Check sheet for the modelled part. Datum: model origin and axes. Units: mm. A direction names the side the tool comes from. Coordinates: 2 decimals unless noted, no trailing zeros. Loops run counter-clockwise (first coordinate to the right, second up) from the corner with the lowest first, then second, coordinate; pieces in that order, holes last.
Autodesk Inventor part; units mm, degrees
ref_plane "YZ Plane" through (0, 0, 0) normal (1, 0, 0) x (0, 1, 0)
ref_plane "XZ Plane" through (0, 0, 0) normal (0, 1, 0) x (-1, 0, 0)
ref_plane "XY Plane" through (0, 0, 0) normal (0, 0, 1) x (1, 0, 0)
sketch "Sketch1" plane through (0, 0, 0) normal (0, 0, 1) x (1, 0, 0)
  arc A0 (37.1972, 10.8951) -> (38.76, 0) centre (0, 0) ccw
  arc A1 (-36.6776, -2.4605) -> (36.6776, -2.4605) centre (0, 0) ccw
  line L0 (-36.76, 0) -> (36.76, 0)
  line L1 (-36.76, 0) -> (37.1972, 0)
  line L2 (36.6776, -2.4605) -> (-36.6776, -2.4605)
  line L3 (-36.76, 0) -> (-38.76, 0)
  line L4 (37.1972, 0) -> (38.76, 0)
  line L5 (0, 0) -> (27.3, 0)
  line L6 (27.3, 0) -> (27.3, -1.7)
  line L7 (27.3, -1.7) -> (0, -1.7)
  line L8 (0, -1.7) -> (0, 0)
  line L9 (-27.3, 0) -> (-27.3, -1.7)
  line L10 (-27.3, -1.7) -> (0, -1.7)
  dimension "d0" = 77.52
  dimension "d1" = 2
extrude "Extrusion1" add sketch "Sketch1" along normal blind 5 contours L3 L0 L9 L10 L7 L6 L1 L4 A0
sketch "Sketch2" plane through (-27.3, -1.7, 0) normal (0, 1, 0) x (1, 0, 0)
  line L0 (54.6, 0) -> (0, 0)
  line L1 (54.6, 0) -> (54.6, -5)
  line L2 (0, 0) -> (0, -5)
  point P0 (27.3, 0)
  point P1 (27.305, -2.3213)
  dimension "d7" = 2.3213
  dimension "d28" = 27.305
hole "Hole1" at (0.005, -1.7, 2.3213) direction (0, -1, 0) diameter 3.81 depth 2.54
sketch "Sketch3" plane through (0, 0, 5) normal (0, 0, 1) x (1, 0, 0)
  arc A0 (2.6516, -28.9347) -> (-2.75, -29.6637) centre (0, -29.6637) ccw
  line L0 (-0.7992, -29.6638) -> (0.7008, -29.6638)
  line L1 (2.6516, -29.6637) -> (2.6516, -38.4638)
  line L2 (2.6516, -38.4638) -> (-2.75, -38.4638)
  line L3 (-2.75, -38.4638) -> (-2.75, -29.6637)
  line L4 (-0.7992, -29.6638) -> (0.7008, -29.6638)
  line L5 (0.7008, -29.6638) -> (0.7008, -33.1638)
  line L6 (0.7008, -33.1638) -> (-0.7992, -33.1638)
  line L7 (-0.7992, -33.1638) -> (-0.7992, -29.6638)
  line L8 (2.6516, -29.6637) -> (2.6516, -28.9347)
  point P0 (0, 0)
  point P1 (-0.0492, -29.6638)
  point P2 (2.6516, -30.3927)
  dimension "d16" = 5.5
  dimension "d17" = 3.5
  dimension "d18" = 1.5
  dimension "d19" = 0.75
extrude "Extrusion2" add sketch "Sketch3" against normal up to surface (5 mm away)
properties part number "Siding Lock"
1) Section check C-C on y = -35. Enter the section's corners in (x, z).
Answer sheet:
outline: (-16.65, 0) - (-11.24, 0) - (-11.24, 5) - (-16.65, 5) - close; (-2.75, 0) - (2.65, 0) - (2.65, 5) - (-2.75, 5) - close; (11.24, 0) - (16.65, 0) - (16.65, 5) - (11.24, 5) - close
2) Section check D-D on z = 2.95. Enter the section's corners in (x, y).
Answer sheet:
outline: (-38.76, 0) arc R38.76 ccw to (38.76, 0) - (27.3, 0) - (27.3, -1.7) - (1.8, -1.7) - (1.8, -2.46) - (36.68, -2.46) arc R36.76 cw to (2.65, -36.66) - (2.65, -28.93) arc R2.75 ccw to (-2.75, -29.66) - (-2.75, -36.66) arc R36.76 cw to (-36.68, -2.46) - (-1.79, -2.46) - (-1.79, -1.7) - (-27.3, -1.7) - (-27.3, 0) - close; hole (-0.8, -33.16) - (0.7, -33.16) - (0.7, -29.66) - (-0.8, -29.66) - close
3) Mould release check, pull along X, two halves, no side actions. Record for faces 5 (the cylindrical face through (-25.835, -26.15, 2.465)), 6 (the flat face through (33, 0, 2)), 7 (the flat face through (0, -29.664, 3)): +X half, -X half, draft (parallel to the pull), parting line (faces both ways), or undercut.
Answer sheet:
face 5: undercut
face 6: draft
face 7: undercut
4) Section check A-A on y = -22.5. Enter the section's corners in (x, z), plus the area to 3 significant figures.
Answer sheet:
outline: (-31.56, 0) - (-29.07, 0) - (-29.07, 5) - (-31.56, 5) - close; (29.07, 0) - (31.56, 0) - (31.56, 5) - (29.07, 5) - close
area: 24.9 mm2
5) Scan lines: line 1 (X direction, y = -32.5, z = 3.65); line 2 (Y direction, x = 2.5, z = 1.65); line 3 (X direction, y = -10, z = 4.5). Record each from-to range of solid material in increasing order.
Answer sheet:
line 1: x = -21.12 to -17.18, -2.75 to -0.8, 0.7 to 2.65, 17.18 to 21.12
line 2: y = -38.68 to -28.52, -2.46 to -1.7
line 3: x = -37.45 to -35.37, 35.37 to 37.45
6) Set-up check for faces 1 (the flat face through (27.3, -1, 2)), 2 (the cylindrical face through (-0.08, -2.09, 0.42)), 3 (the flat face through (2.652, -33, 3)), 4 (the flat face through (-33, 0, 2)): record each of +Z, -Z, +X, -X, +Y, -Y from which the full face is reachable in a straight line by a thin tool's end or side.
Answer sheet:
face 1: +Z, -Z, +Y
face 2: +Y
face 3: +Z, -Z
face 4: +Z, -Z, +X, -X, +Y
7) Depth check by flat-ended pin: pin 1 (1.1 mm diameter, centred on y = -31, z = 2, fed in from -X); pin 2 (3 mm diameter, centred on y = -26, z = 1, fed in from +X); pin 3 (3 mm diameter, centred on x = 4, z = 0.5, fed in from -Y); pin 4 (10 mm diameter, centred on x = 13, y = -8, fed in from -Z). Enter the tip coordinate at first touch or a pass-through.
Answer sheet:
pin 1: stops at x = -23.98
pin 2: stops at x = 30.03
pin 3: stops at y = -38.68
pin 4: passes through
8) Section check B-B on x = -31. Enter the section's corners in (y, z), plus the area to 3 significant figures.
Answer sheet:
outline: (-23.27, 0) - (-19.76, 0) - (-19.76, 5) - (-23.27, 5) - close; (-2.46, 0) - (0, 0) - (0, 5) - (-2.46, 5) - close
area: 29.9 mm2
